The model under review builds one solid part; all positions refer to its coordinate system, in mm. A direction names the side the tool comes from. Coordinates: 2 decimals unless noted, no trailing zeros. Order: outer loops, then holes, each group sorted by start corner. A loop starts at its lowest first (then second) coordinate and runs counter-clockwise, first axis right, second up.
from build123d import *

# Parameters (mm, degrees)
F0_W     = 7.332219354
F0_H     = 16.389713157
F1_DEPTH = 3.556


with BuildPart() as f1:
    # F0 (on Front) → F1 (new body)
    with BuildSketch(Plane.XZ):
        with Locations((31.0518859964, 5.022654077)):
            Rectangle(F0_W, F0_H)
        with Locations((31.0518859964, -11.3670590799)):
            Rectangle(F0_W, F0_H)
        with BuildLine():
            Line((25.3776218742, -3.1722025014), (25.3776218742, -27.8178208713))
            ThreePointArc((25.3776218742, -27.8178208713), (31.379030254, -23.0253955717), (36.7261501186, -28.5383396079))
            Line((36.7261501186, -28.5383396079), (36.7261501186, -3.1722025014))
            Line((36.7261501186, -3.1722025014), (34.7179956734, -3.1722025014))
            Line((34.7179956734, -3.1722025014), (34.7179956734, -19.5619156584))
            Line((34.7179956734, -19.5619156584), (27.3857763194, -19.5619156584))
            Line((27.3857763194, -19.5619156584), (27.3857763194, -3.1722025014))
            Line((27.3857763194, -3.1722025014), (25.3776218742, -3.1722025014))
        make_face()
        with BuildLine():
            ThreePointArc((34.3040495539, -28.9137765537), (31.0170948505, -32.0183687355), (27.7301401472, -28.9137765537))
            Line((27.7301401472, -28.9137765537), (25.3776218742, -28.9137765537))
            Line((25.3776218742, -28.9137765537), (25.3776218742, -27.8178208713))
            ThreePointArc((25.3776218742, -27.8178208713), (30.4680136742, -34.4117471456), (36.7261501186, -28.9137765537))
            Line((36.7261501186, -28.9137765537), (34.3040495539, -28.9137765537))
        make_face()
        with BuildLine():
            ThreePointArc((27.7301401472, -28.9137765537), (30.9231974181, -25.4350866863), (34.3094055053, -28.7260580808))
            ThreePointArc((34.3094055053, -28.7260580808), (34.308066245, -28.8199555132), (34.3040495539, -28.9137765537))
            Line((34.3040495539, -28.9137765537), (36.7261501186, -28.9137765537))
            Line((36.7261501186, -28.9137765537), (36.7261501186, -28.5383396079))
            ThreePointArc((36.7261501186, -28.5383396079), (31.379030254, -23.0253955717), (25.3776218742, -27.8178208713))
            Line((25.3776218742, -27.8178208713), (25.3776218742, -28.9137765537))
            Line((25.3776218742, -28.9137765537), (27.7301401472, -28.9137765537))
        make_face()
    extrude(amount=F1_DEPTH)


solid = f1.part
(1) Insertion check: pin 1 Ø1 at (x, y) = (35.5, -2) entering from +Z; pin 2 Ø1.5 at (x, y) = (27.5, -1) entering from -Z. Each pin has a flat end and moves straight along its axis. Give the tip position at first contact, or say it passes through.
(2) Consider section B-B (y = -3). Give the boundary of the cut face in (x, z), then the cut area to 3 significant figures.
(3) Tool access review of faces 1 (the face through (27.386, -2, 5)), 2 (the face through (34.718, -2, 5)), 3 (the face through (31, -3.556, -10)): name each direction out of +Z, -Z, +X, -X, +Y, -Y from which nothing blocks a thin tool from reaching the whole face with its end or side.
(4) Consider section A-A (x = 32.5). Give the boundary of the cut face in (y, z).
(5) Consider section C-C (z = -31). Give the boundary of the cut face in (x, y), then the cut area to 3 significant figures.
(6) Wall thickness on line 1 (X direction, y = -2.65, z = -29); line 2 (Z direction, x = 31, y = -2.05); line 3 (X direction, y = -1.9, z = -4): over which ranges is each line inside the solid? List them lowest first.
(7) Consider section D-D (z = 4.5). Give the boundary of the cut face in (x, y).
Findings:
1. pin 1: stops at z = -3.17
1. pin 2: stops at z = -33.72
2. outline: (25.38, -27.82) arc R5.71 ccw (long way) to (36.73, -28.91) - (36.73, -3.17) - (34.72, -3.17) - (34.72, 13.22) - (27.39, 13.22) - (27.39, -3.17) - (25.38, -3.17) - close; hole circle Ø6.58 at (31.02, -28.73)
2. area: 427 mm2
3. face 1: +Z, -X, +Y, -Y
3. face 2: +Z, +X, +Y, -Y
3. face 3: +Z, -Z, +X, -X, -Y
4. outline: (-3.56, -34.24) - (0, -34.24) - (0, -31.67) - (-3.56, -31.67) - close; (-3.56, -25.79) - (0, -25.79) - (0, 13.22) - (-3.56, 13.22) - close
5. outline: (25.78, -3.56) - (28.64, -3.56) - (28.64, 0) - (25.78, 0) - close; (33.4, -3.56) - (36.26, -3.56) - (36.26, 0) - (33.4, 0) - close
5. area: 20.3 mm2
6. line 1: x = 25.31 to 27.74, 34.3 to 36.72
6. line 2: z = -34.44 to -32.02, -25.43 to 13.22
6. line 3: x = 25.38 to 36.73
7. outline: (27.39, -3.56) - (34.72, -3.56) - (34.72, 0) - (27.39, 0) - close
